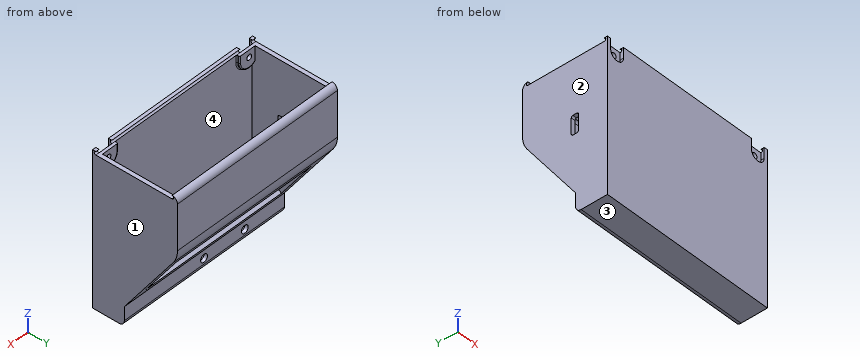
from build123d import *

# Parameters (mm, degrees)
BOSS_EXTRUDE1_DEPTH = 85
CUT_EXTRUDE1_START  = 1.95
CUT_EXTRUDE1_DEPTH  = 81.1
CUT_EXTRUDE5_REACH  = 51.22
SKETCH5_W           = 72
SKETCH5_H           = 25
SKETCH5_3_W         = 78
SKETCH5_3_H         = 31
SKETCH5_3_W_2       = 72
SKETCH5_3_H_2       = 25
BOSS_EXTRUDE3_DEPTH = 5.6
SKETCH6_R           = 1.825
CUT_EXTRUDE6_DEPTH  = 13.6
CUT_EXTRUDE7_REACH  = 87
SKETCH12_R          = 1.5
CUT_EXTRUDE10_DEPTH = 1.6
SKETCH12_5_R        = 1.5
SKETCH12_5_R_2      = 1.3
BOSS_EXTRUDE7_DEPTH = 3
SKETCH12_6_R        = 1.5
SKETCH12_6_R_2      = 1.3
CUT_EXTRUDE11_DEPTH = 1.6
CUT_EXTRUDE8_REACH  = 87
FILLET2_R           = 0.5


with BuildPart() as part:
    # Sketch1 → Boss-Extrude1 (new body)
    with BuildSketch(Plane(origin=(0, 0, 0), x_dir=(0, 0, -1), z_dir=(1, 0, 0))):
        with BuildLine():
            Line((-22.930528586, 36.4), (-22.930528586, -1.6))
            Line((-22.930528586, -1.6), (50.269471414, -1.6))
            Line((50.269471414, -1.6), (50.269471414, 11))
            ThreePointArc((50.269471414, 11), (49.507949045, 12.838477631), (47.669471414, 13.6))
            Line((47.669471414, 13.6), (41.173949476, 13.6))
            Line((41.173949476, 13.6), (7.895010815, 36.902163714))
            ThreePointArc((7.895010815, 36.902163714), (4.729711428, 38.463116629), (1.241524153, 39))
            Line((1.241524153, 39), (-20.330528586, 39))
            ThreePointArc((-20.330528586, 39), (-22.169006218, 38.238477631), (-22.930528586, 36.4))
        make_face()
    extrude(amount=BOSS_EXTRUDE1_DEPTH)

    # Sketch1_3 → Cut-Extrude1 (cut)
    with BuildSketch(Plane(origin=(0, 0, 0), x_dir=(0, 0, -1), z_dir=(1, 0, 0)).offset(CUT_EXTRUDE1_START)):
        with BuildLine():
            Line((48.669471414, 0), (48.669471414, 11))
            ThreePointArc((48.669471414, 11), (48.376578195, 11.707106781), (47.669471414, 12))
            Line((47.669471414, 12), (40.669471414, 12))
            Line((40.669471414, 12), (6.977288517, 35.591520443))
            ThreePointArc((6.977288517, 35.591520443), (4.248582149, 36.937169507), (1.241524153, 37.4))
            Line((1.241524153, 37.4), (-20.330528586, 37.4))
            ThreePointArc((-20.330528586, 37.4), (-21.037635368, 37.107106781), (-21.330528586, 36.4))
            Line((-21.330528586, 36.4), (-21.330528586, 0))
            Line((-21.330528586, 0), (48.669471414, 0))
        make_face()
    extrude(amount=CUT_EXTRUDE1_DEPTH, mode=Mode.SUBTRACT)

    # Sketch5 → Cut-Extrude5 (cut, up to next)
    with BuildSketch(Plane(origin=(0, 28.47116522, -19.935724509), x_dir=(1, 0, 0), z_dir=(0, 0.819152044, -0.573576436)), mode=Mode.PRIVATE) as cut_extrude5_sk1:
        with Locations((42.5, 5.614044021)):
            Rectangle(SKETCH5_W, SKETCH5_H)
    cut_extrude5_tool1 = extrude(cut_extrude5_sk1.sketch, amount=-CUT_EXTRUDE5_REACH, mode=Mode.PRIVATE) & part.part
    add(cut_extrude5_tool1.solids().sort_by_distance((42.5, 25.251082, -24.53448))[0], mode=Mode.SUBTRACT)

    # Sketch5_3 → Boss-Extrude3 (add)
    with BuildSketch(Plane(origin=(0, 28.47116522, -19.935724509), x_dir=(1, 0, 0), z_dir=(0, 0.819152044, -0.573576436))):
        with Locations((42.5, 5.614044021)):
            Rectangle(SKETCH5_3_W, SKETCH5_3_H)
        with Locations((42.5, 5.614044021)):
            Rectangle(SKETCH5_3_W_2, SKETCH5_3_H_2, mode=Mode.SUBTRACT)
    extrude(amount=-BOSS_EXTRUDE3_DEPTH)

    # Sketch6 → Cut-Extrude6 (cut)
    with BuildSketch(Plane(origin=(0, 13.6, 0), x_dir=(1, 0, 0), z_dir=(0, 1, 0))):
        with Locations((21, 44.969471414)):
            Circle(SKETCH6_R)
        with Locations((42.65, 44.969471414)):
            Circle(SKETCH6_R)
    extrude(amount=-CUT_EXTRUDE6_DEPTH, mode=Mode.SUBTRACT)

    # Sketch7 → Cut-Extrude7 (cut, up to next)
    with BuildSketch(Plane.ZY, mode=Mode.PRIVATE) as cut_extrude7_sk1:
        with BuildLine():
            Line((-12.869471414, 15.725), (-5.319471414, 15.725))
            ThreePointArc((-5.319471414, 15.725), (-4.753785989, 15.490685425), (-4.519471414, 14.925))
            Line((-4.519471414, 14.925), (-4.519471414, 13.075))
            ThreePointArc((-4.519471414, 13.075), (-4.753785989, 12.509314575), (-5.319471414, 12.275))
            Line((-5.319471414, 12.275), (-12.869471414, 12.275))
            ThreePointArc((-12.869471414, 12.275), (-13.435156838, 12.509314575), (-13.669471414, 13.075))
            Line((-13.669471414, 13.075), (-13.669471414, 14.925))
            ThreePointArc((-13.669471414, 14.925), (-13.435156838, 15.490685425), (-12.869471414, 15.725))
        make_face()
    cut_extrude7_tool1 = extrude(cut_extrude7_sk1.sketch, amount=-CUT_EXTRUDE7_REACH, mode=Mode.PRIVATE) & part.part
    add(cut_extrude7_tool1.solids().sort_by_distance((0, 14, -9.094471))[0], mode=Mode.SUBTRACT)

    # Sketch12 → Cut-Extrude10 (cut)
    with BuildSketch(Plane.XZ.offset(1.6)):
        with Locations((79.9, 17.930528586)):
            Circle(SKETCH12_R)
        with Locations((5.1, 17.930528586)):
            Circle(SKETCH12_R)
    extrude(amount=-CUT_EXTRUDE10_DEPTH, mode=Mode.SUBTRACT)

    # Sketch12_5 → Boss-Extrude7 (add)
    with BuildSketch(Plane.XZ.offset(1.6)):
        with BuildLine():
            ThreePointArc((83.3, 17.930528586), (79.9, 14.530528586), (76.5, 17.930528586))
            Line((76.5, 17.930528586), (76.5, 22.930528586))
            Line((76.5, 22.930528586), (74.85, 22.930528586))
            Line((74.85, 22.930528586), (74.85, 17.930528586))
            ThreePointArc((74.85, 17.930528586), (79.9, 12.880528586), (84.95, 17.930528586))
            Line((84.95, 17.930528586), (84.95, 22.930528586))
            Line((84.95, 22.930528586), (83.3, 22.930528586))
            Line((83.3, 22.930528586), (83.3, 17.930528586))
        make_face()
        with BuildLine():
            Line((76.5, 22.930528586), (76.5, 17.930528586))
            ThreePointArc((76.5, 17.930528586), (79.9, 14.530528586), (83.3, 17.930528586))
            Line((83.3, 17.930528586), (83.3, 22.930528586))
            Line((83.3, 22.930528586), (76.5, 22.930528586))
        make_face()
        with Locations((79.9, 17.930528586)):
            Circle(SKETCH12_5_R, mode=Mode.SUBTRACT)
        with Locations((79.9, 17.930528586)):
            Circle(SKETCH12_5_R)
        with Locations((79.9, 17.930528586)):
            Circle(SKETCH12_5_R_2, mode=Mode.SUBTRACT)
        with BuildLine():
            Line((10.15, 17.930528586), (10.15, 22.930528586))
            Line((10.15, 22.930528586), (8.5, 22.930528586))
            Line((8.5, 22.930528586), (8.5, 17.930528586))
            ThreePointArc((8.5, 17.930528586), (5.1, 14.530528586), (1.7, 17.930528586))
            Line((1.7, 17.930528586), (1.7, 22.930528586))
            Line((1.7, 22.930528586), (0.05, 22.930528586))
            Line((0.05, 22.930528586), (0.05, 17.930528586))
            ThreePointArc((0.05, 17.930528586), (5.1, 12.880528586), (10.15, 17.930528586))
        make_face()
        with BuildLine():
            Line((8.5, 17.930528586), (8.5, 22.930528586))
            Line((8.5, 22.930528586), (1.7, 22.930528586))
            Line((1.7, 22.930528586), (1.7, 17.930528586))
            ThreePointArc((1.7, 17.930528586), (5.1, 14.530528586), (8.5, 17.930528586))
        make_face()
        with Locations((5.1, 17.930528586)):
            Circle(SKETCH12_5_R, mode=Mode.SUBTRACT)
        with Locations((5.1, 17.930528586)):
            Circle(SKETCH12_5_R)
        with Locations((5.1, 17.930528586)):
            Circle(SKETCH12_5_R_2, mode=Mode.SUBTRACT)
    extrude(amount=-BOSS_EXTRUDE7_DEPTH)

    # Sketch12_6 → Cut-Extrude11 (cut)
    with BuildSketch(Plane.XZ.offset(1.6)):
        with BuildLine():
            Line((8.5, 17.930528586), (8.5, 22.930528586))
            Line((8.5, 22.930528586), (1.7, 22.930528586))
            Line((1.7, 22.930528586), (1.7, 17.930528586))
            ThreePointArc((1.7, 17.930528586), (5.1, 14.530528586), (8.5, 17.930528586))
        make_face()
        with Locations((5.1, 17.930528586)):
            Circle(SKETCH12_6_R, mode=Mode.SUBTRACT)
        with BuildLine():
            Line((76.5, 22.930528586), (76.5, 17.930528586))
            ThreePointArc((76.5, 17.930528586), (79.9, 14.530528586), (83.3, 17.930528586))
            Line((83.3, 17.930528586), (83.3, 22.930528586))
            Line((83.3, 22.930528586), (76.5, 22.930528586))
        make_face()
        with Locations((79.9, 17.930528586)):
            Circle(SKETCH12_6_R, mode=Mode.SUBTRACT)
        with Locations((79.9, 17.930528586)):
            Circle(SKETCH12_6_R)
        with Locations((79.9, 17.930528586)):
            Circle(SKETCH12_6_R_2, mode=Mode.SUBTRACT)
        with Locations((5.1, 17.930528586)):
            Circle(SKETCH12_6_R)
        with Locations((5.1, 17.930528586)):
            Circle(SKETCH12_6_R_2, mode=Mode.SUBTRACT)
    extrude(amount=-CUT_EXTRUDE11_DEPTH, mode=Mode.SUBTRACT)

    # Sketch9 → Cut-Extrude8 (cut, up to next)
    with BuildSketch(Plane(origin=(0, 0, 0), x_dir=(0, 0, -1), z_dir=(1, 0, 0)), mode=Mode.PRIVATE) as cut_extrude8_sk1:
        with BuildLine():
            Line((-21.330528586, 35.411275227), (-21.330528586, 0))
            ThreePointArc((-21.330528586, 0), (-22.1361662, -0.794362387), (-22.930528586, 0.011275227))
            Line((-22.930528586, 0.011275227), (-22.930528586, 36.4))
            ThreePointArc((-22.930528586, 36.4), (-22.130528586, 37.2), (-21.330528586, 36.4))
            Line((-21.330528586, 36.4), (-21.330528586, 35.411275227))
        make_face()
    cut_extrude8_tool1 = extrude(cut_extrude8_sk1.sketch, amount=CUT_EXTRUDE8_REACH, mode=Mode.PRIVATE) & part.part
    add(cut_extrude8_tool1.solids().sort_by_distance((0, 18.202803, 22.130529))[0], mode=Mode.SUBTRACT)

    # Fillet2
    fillet2_edges = [part.edges().sort_by_distance(p)[0] for p in [
        (74.85, 0, 19.630528586),
        (77.709680389, 0, 13.380253869),
        (77.709680389, 1.4, 13.380253869),
        (74.85, 1.4, 19.630528586),
        (7.290319611, 0, 13.380253869),
        (10.15, 1.4, 19.630528586),
        (10.15, 0, 19.630528586),
        (7.290319611, 1.4, 13.380253869),
    ]]
    fillet(fillet2_edges, radius=FILLET2_R)


solid = part.part
Geometry: final body of the model. Coordinates: model frame, mm. Face numbers are marked on the shaded views. Give positions to 0.01 mm unless a question says otherwise; leave off trailing zeros. Loops run counter-clockwise (first coordinate to the right, second up) from the corner with the lowest first, then second, coordinate; pieces in that order, holes last. Notation, with made-up numbers: (87.25, 59) - (112.25, 59) arc R29 cw to (112.25, 85) - close; hole circle Ø8 at (-36.5, 18.5). An arc over 180 degrees is marked (long way). One line per question, with ' | ' between items. Start each with the question number.
(1) Section query B-B on z = 10. Return loops of the section in (x, y), then the cut area to 3 significant figures.
(2) Ray query, line 1 (Z direction, x = 5.1, y = 0.8); line 2 (X direction, y = 21.5, z = -25); line 3 (X direction, y = 4, z = -42). Return the intervals inside material, ascending. Write a range as from..to.
(3) Pull-direction query (X, two-part tool) for the marked faces 1, 2, 3 and 4; classes: released by +X, released by -X, zero draft, split by the parting line, or undercut.
(4) Section query C-C on x = 42.65. Count the separate pieces of the cut face and the enclosed holes in it, then the cut area to 3 significant figures.
(5) Section query D-D on z = -17.5. Return loops of the section in (x, y), then the cut area to 3 significant figures.
(6) Contact query for flat-ended pins moving along their axis: pin 1 (8 mm diameter, centred on x = 63.5, y = 21.5, fed in from -Z); pin 2 (2 mm diameter, centred on x = 36, y = 29, fed in from -Z); pin 3 (4.5 mm diameter, centred on x = 21, z = -44.97, fed in from +Y). Output: stop coordinate, or through.
The answers:
1) outline: (0, -1.6) - (85, -1.6) - (85, 39) - (0, 39) - close; hole (1.95, 0) - (83.05, 0) - (83.05, 37.4) - (1.95, 37.4) - close | area: 418 mm2
2) line 1: -50.27..-48.67, 12.88..16.63, 19.23..21.33 | line 2: 0..1.95, 3.5..6.5, 78.5..81.5, 83.05..85 | line 3: 0..1.95, 83.05..85
3) face 1: released by +X | face 2: released by -X | face 3: zero draft | face 4: undercut
4) separate pieces: 3 | enclosed holes: 0 | area: 241 mm2
5) outline: (0, -1.6) - (85, -1.6) - (85, 30.18) - (78.5, 30.18) - (78.5, 23.34) - (81.5, 23.34) - (81.5, 28.22) - (83.05, 28.22) - (83.05, 0) - (1.95, 0) - (1.95, 28.22) - (3.5, 28.22) - (3.5, 23.34) - (6.5, 23.34) - (6.5, 30.18) - (0, 30.18) - close | area: 301 mm2
6) pin 1: z = -35.6 | pin 2: z = -12.6 | pin 3: y = 13.6
